Study the drawing (mm; zero at the part's minimum x, y, z) and answer. Coordinates: 2 decimals unless noted, no trailing zeros. Loops run counter-clockwise (first coordinate to the right, second up) from the corner with the lowest first, then second, coordinate; pieces in that order, holes last. Notation, with made-up numbers: (81.5, 14) - (108.5, 14) arc R26 cw to (108.5, 43) - close; hole circle Ø3 at (-9, 65.25). An arc over 180 degrees is marked (long way). Put each result on its own line as item: value.
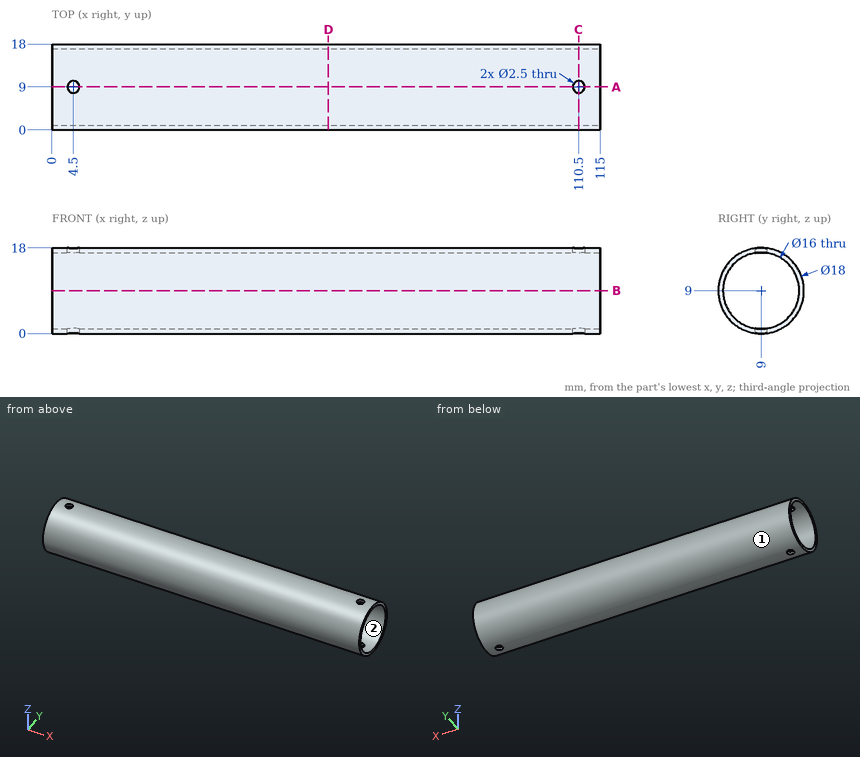
1) Straight lines are drawn through the part: L1, parallel to Z at x = 74, y = 8.5; L2, parallel to Y at x = 47, z = 2.75; L3, parallel to Y at x = 40.5, z = 8.75. For each, find the intervals that lie inside material, in ascending order. Write a range as [from, to].
Found:
L1: z = [0.01, 1.02], [16.98, 17.99]
L2: y = [2.52, 4.01], [13.99, 15.48]
L3: y = [0, 1], [17, 18]
2) Each of these flat-tipped pins is pushed along its axis until it touches: pin 1 (5 mm diameter, centred on x = 92.5, z = 4, fed in from -Y); pin 2 (10 mm diameter, centred on x = 21, y = 2.5, fed in from -Z); pin 3 (1.5 mm diameter, centred on x = 78, y = 15.5, fed in from -Z). Where does it stop, or does it pass through?
Found:
pin 1: stops at y = 0.35
pin 2: stops at z = 0.13
pin 3: stops at z = 2.08
3) The part is cut by section B-B (z = 9). Give the vertices of the cut face in (x, y), and give its area (3 significant figures).
Found:
outline: (0, 0) - (115, 0) - (115, 1) - (0, 1) - close; (0, 17) - (115, 17) - (115, 18) - (0, 18) - close
area: 230 mm^2
4) For a pull along Z with two mould halves and no side action, classify the marked faces 1 and 2 as pulls with the +Z half, pulls with the -Z half, needs draft (parallel to the pull), parting line crosses it, or undercut.
Found:
face 1: parting line crosses it
face 2: undercut
5) The part is cut by section C-C (x = 110.5). Give the vertices of the cut face in (y, z).
Found:
outline: (7.75, 0.09) - (7.75, 1.1) arc R8 cw to (7.75, 16.9) - (7.75, 17.91) arc R9 ccw to start; (10.25, 0.09) arc R9 ccw to (10.25, 17.91) - (10.25, 16.9) arc R8 cw to (10.25, 1.1) - close
6) The part is cut by section D-D (x = 58). Give the vertices of the cut face in (y, z).
Found:
outline: circle Ø18 at (9, 9); hole circle Ø16 at (9, 9)
7) The part is cut by section A-A (y = 9). Give the vertices of the cut face in (x, z).
Found:
outline: (0, 0) - (3.25, 0) - (3.25, 1) - (0, 1) - close; (0, 17) - (3.25, 17) - (3.25, 18) - (0, 18) - close; (5.75, 0) - (109.25, 0) - (109.25, 1) - (5.75, 1) - close; (5.75, 17) - (109.25, 17) - (109.25, 18) - (5.75, 18) - close; (111.75, 0) - (115, 0) - (115, 1) - (111.75, 1) - close; (111.75, 17) - (115, 17) - (115, 18) - (111.75, 18) - close
